Geometry check sheet. Reference: the model listing, model coordinates, mm. Face numbers are marked on the shaded views. A direction names the side the tool comes from. Round coordinates to 2 decimals unless told otherwise and drop trailing zeros. Loops run counter-clockwise (first coordinate to the right, second up) from the corner with the lowest first, then second, coordinate; pieces in that order, holes last. Notation, with made-up numbers: (-27, 20) - (-5, 20) arc R20 ccw to (-5, 33) - close; hole circle Ø9 at (8, -35). An arc over 180 degrees is marked (long way). Answer in a Markdown table with one row per item. Add a question column.
```python
from build123d import *

# Parameters (mm, degrees)
F0_R     = 25
F1_DEPTH = 125
F0_W     = 150
F0_H     = 65
F2_DEPTH = 35
F3_R     = 10
F4_DEPTH = 100.001


with BuildPart() as f1:
    # F0 (on Top) → F1 (new body)
    with BuildSketch(Plane.XY):
        with BuildLine():
            Line((125, 0), (-125, 0))
            Line((-125, 0), (-125, -35))
            Line((-125, -35), (25, -35))
            Line((25, -35), (25, -100))
            ThreePointArc((25, -100), (75, -150), (125, -100))
            Line((125, -100), (125, 0))
        make_face()
        with Locations((75, -100)):
            Circle(F0_R, mode=Mode.SUBTRACT)
    extrude(amount=F1_DEPTH)

    # F0 (on Top) → F2 (join)
    with BuildSketch(Plane.XY):
        with Locations((-50, -67.5)):
            Rectangle(F0_W, F0_H)
    extrude(amount=F2_DEPTH)

    # F3 (on face) → F4 (cut, through all)
    with BuildSketch(Plane.XZ.offset(100)):
        with Locations((-87.5, 17.5)):
            Circle(F3_R)
        with Locations((-12.5, 17.5)):
            Circle(F3_R)
    extrude(amount=-F4_DEPTH, mode=Mode.SUBTRACT)


solid = f1.part
```
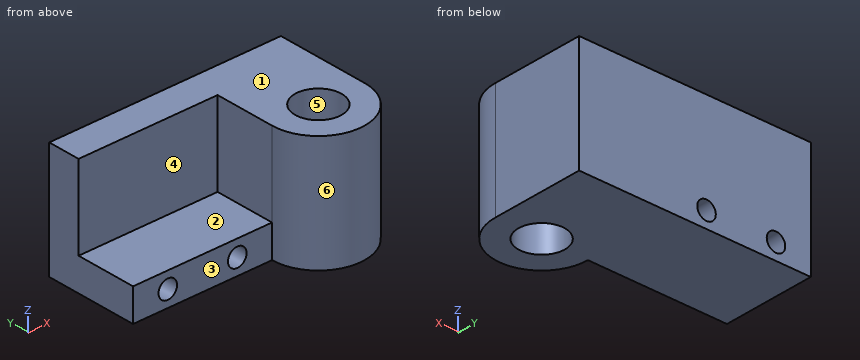
Q1. Set-up check for the marked faces 1, 2 and 3: record each of +Z, -Z, +X, -X, +Y, -Y from which the full face is reachable in a straight line by a thin tool's end or side.
Q2. Cross-section at D-D, the plane z = 63. Enter the section's corners in (x, y), plus the area to 3 significant figures.
Q3. Scan lines: line 1 (X direction, y = -50, z = 17); line 2 (Y direction, x = 75, z = 71); line 3 (Z direction, x = -87, y = -27). Record each from-to range of solid material in increasing order. Write a range as from..to.
Q4. Cross-section at A-A, the plane z = 17.5. Enter the section's corners in (x, y), plus the area to 3 significant figures.
Q5. Cross-section at B-B, the plane x = -87.5. Enter the section's corners in (y, z), plus the area to 3 significant figures.
Q6. Depth check by flat-ended pin: P1, Ø8, axis at x = -4.5, z = 87, coming from the -Y side; P2, Ø3, axis at y = -101, z = 80.5, coming from the -X side; P3, Ø1.5, axis at x = 81.5, z = 47, coming from the -Y side. Enter the tip coordinate at first touch or a pass-through.
Q7. Cross-section at C-C, the plane y = -81. Enter the section's corners in (x, z), plus the area to 3 significant figures.
Q8. Release check for a two-part mould opening along X. For the marked faces 4, 5 and 6 record: +X half, -X half, draft (parallel to the pull), parting line (faces both ways), or undercut.
Check sheet entries:
| question | item | result |
|---|---|---|
| 1 | face 1 | +Z, +X, -X, +Y, -Y |
| 1 | face 2 | +Z, -X, -Y |
| 1 | face 3 | +Z, -Z, -X, -Y |
| 2 | outline | (-125, -35) - (25, -35) - (25, -100) arc R50 ccw to (125, -100) - (125, 0) - (-125, 0) - close; hole circle Ø50 at (75, -100) |
| 2 | area | 17,200 mm² |
| 3 | line 1 | -125..-97.49, -77.51..-22.49, -2.51..125 |
| 3 | line 2 | -150..-125, -75..0 |
| 3 | line 3 | 0..7.51, 27.49..125 |
| 4 | outline | (-125, -100) - (-97.5, -100) - (-97.5, 0) - (-125, 0) - close; (-77.5, -100) - (-22.5, -100) - (-22.5, 0) - (-77.5, 0) - close; (-2.5, -100) - (25, -100) arc R50 ccw to (125, -100) - (125, 0) - (-2.5, 0) - close; hole circle Ø50 at (75, -100) |
| 4 | area | 23,000 mm² |
| 5 | outline | (-100, 0) - (0, 0) - (0, 7.5) - (-100, 7.5) - close; (-100, 27.5) - (0, 27.5) - (0, 125) - (-35, 125) - (-35, 35) - (-100, 35) - close |
| 5 | area | 4,650 mm² |
| 6 | P1 | y = -35 |
| 6 | P2 | x = 25 |
| 6 | P3 | y = -149.67 |
| 7 | outline | (-125, 0) - (58.75, 0) - (58.75, 125) - (25, 125) - (25, 35) - (-125, 35) - close; (91.25, 0) - (125, 0) - (125, 125) - (91.25, 125) - close; hole circle Ø20 at (-87.5, 17.5); hole circle Ø20 at (-12.5, 17.5) |
| 7 | area | 13,100 mm² |
| 8 | face 4 | draft |
| 8 | face 5 | undercut |
| 8 | face 6 | parting line |
